```python
from build123d import *

# Parameters (mm, degrees)
F0_R            = 25.5
F0_R_2          = 23.5
F1_DEPTH        = 1050
F3_W            = 5
F3_H            = 20
F3_W_2          = 20
F3_H_2          = 5
F4_COPIES_COUNT = 4
F5_R            = 5.25
F6_DEPTH        = 150.001
F6_DEPTH_BACK   = 150.001


# Not quite as in the source:
# - a pattern or mirror of a feature is missing from the dataset's text; its kind, count and spacing are read off the source's solid


with BuildPart() as f1:
    # F0 (on Top) → F1 (new body)
    with BuildSketch(Plane.XY):
        Circle(F0_R)
        Circle(F0_R_2, mode=Mode.SUBTRACT)
    extrude(amount=F1_DEPTH)

    # F3 (on offset) → F4 (join, up to the next surface of F1)
    with BuildSketch(Plane.YZ.offset(150)):
        with Locations((0, 10)):
            Rectangle(F3_W, F3_H)
        with Locations((0, 202.5)):
            Rectangle(F3_W_2, F3_H_2)
    f4 = extrude(until=Until.NEXT, dir=(-1, 0, 0))

    # F4_copies: F4 ×4 about axis
    f4_copies_axis = Axis((0, 0, 0), (0, 0, 1))
    for i in range(1, F4_COPIES_COUNT):
        add(f4.rotate(f4_copies_axis, i * 360 / F4_COPIES_COUNT))

    # F5 (on Front) → F6 (cut, two sides)
    with BuildSketch(Plane.XZ) as f6_sk:
        with Locations((0, 600)):
            Circle(F5_R)
        with Locations((0, 700)):
            Circle(F5_R)
        with Locations((0, 800)):
            Circle(F5_R)
        with Locations((0, 900)):
            Circle(F5_R)
    extrude(amount=-F6_DEPTH, mode=Mode.SUBTRACT)
    extrude(f6_sk.sketch, amount=F6_DEPTH_BACK, mode=Mode.SUBTRACT)


solid = f1.part
```
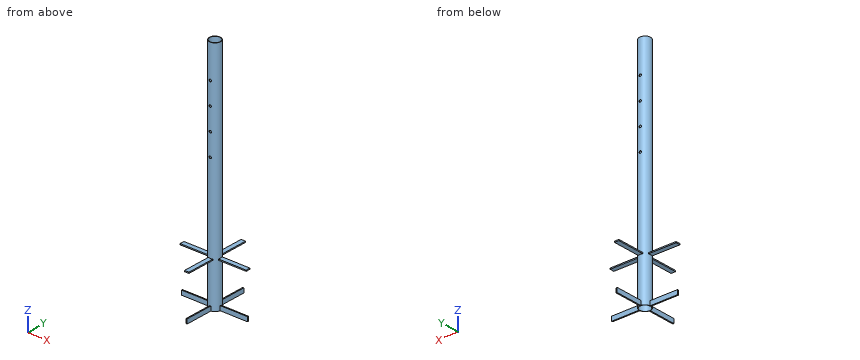
Check sheet for the modelled part. Datum: model origin and axes. Units: mm. Round coordinates to 2 decimals unless told otherwise and drop trailing zeros. Order: outer loops, then holes, each group sorted by start corner. A loop starts at its lowest first (then second) coordinate and runs counter-clockwise, first axis right, second up.
1) Section check A-A (x = 78). Record the boundary of the cut face in (y, z).
2) Scan lines: line 1 (Z direction, x = 0, y = 24); line 2 (Y direction, x = 13, z = 772); line 3 (Y direction, x = 21.5, z = 802). Record each from-to range of solid material in increasing order.
3) Go/stop test with flat-tipped pins: pin 1 Ø1.5 at (x, z) = (86.5, 202) entering from +Y; pin 2 Ø9.5 at (x, z) = (0, 900) entering from -Y; pin 3 Ø10 at (y, z) = (71, 8) entering from -X; pin 4 Ø1.5 at (x, y) = (0.5, 94) entering from +Z. Record where each tip stops, or that it passes through.
4) Section check C-C (z = 639). Record the boundary of the cut face in (x, y).
Result:
1. outline: (-10, 200) - (10, 200) - (10, 205) - (-10, 205) - close; (-2.5, 0) - (2.5, 0) - (2.5, 20) - (-2.5, 20) - close
2. line 1: z = 0 to 594.75, 605.25 to 694.75, 705.25 to 794.75, 805.25 to 894.75, 905.25 to 1050
2. line 2: y = -21.94 to -19.58, 19.58 to 21.94
2. line 3: y = -13.71 to -9.49, 9.49 to 13.71
3. pin 1: stops at y = 10
3. pin 2: passes through
3. pin 3: stops at x = -2.5
3. pin 4: stops at z = 205
4. outline: circle Ø51 at (0, 0); hole circle Ø47 at (0, 0)
